```python
from build123d import *

# Parameters (mm, degrees)
SK_OUTPUT_PLATE_W        = 120.5
SK_OUTPUT_PLATE_H        = 93.5
SK_OUTPUT_PLATE_R        = 1.7
SK_OUTPUT_PLATE_R_2      = 5
OUTPUT_PLATE_DEPTH       = 5
SK_PITCH_PILOT_RECESS_R  = 15.15
PITCH_PILOT_RECESS_DEPTH = 2.2
SK_REAR_PLATE_W          = 93.5
SK_REAR_PLATE_H          = 86.75
SK_REAR_PLATE_R          = 8
SK_REAR_PLATE_R_2        = 1.7
REAR_PLATE_DEPTH         = 5
SK_TOP_PLATE_W           = 45.5
SK_TOP_PLATE_H           = 86.75
TOP_PLATE_DEPTH          = 5
SK_BOTTOM_PLATE_W        = 45.5
SK_BOTTOM_PLATE_H        = 86.75
BOTTOM_PLATE_DEPTH       = 5


with BuildPart() as part:
    # SK_Output_Plate → Output_Plate (new body)
    with BuildSketch(Plane(origin=(0, 0, 0), x_dir=(1, 0, 0), z_dir=(0, 1, 0))):
        with Locations((-30.25, 0)):
            Rectangle(SK_OUTPUT_PLATE_W, SK_OUTPUT_PLATE_H)
        with Locations(Location((20, 0, 0), (0, 0, 270))):
            Circle(SK_OUTPUT_PLATE_R, mode=Mode.SUBTRACT)
        with Locations(Location((10, 17.320508076, 0), (0, 0, 270))):
            Circle(SK_OUTPUT_PLATE_R, mode=Mode.SUBTRACT)
        with Locations(Location((-10, 17.320508076, 0), (0, 0, 270))):
            Circle(SK_OUTPUT_PLATE_R, mode=Mode.SUBTRACT)
        with Locations(Location((-20, 0, 0), (0, 0, 270))):
            Circle(SK_OUTPUT_PLATE_R, mode=Mode.SUBTRACT)
        with Locations(Location((-10, -17.320508076, 0), (0, 0, 270))):
            Circle(SK_OUTPUT_PLATE_R, mode=Mode.SUBTRACT)
        with Locations(Location((10, -17.320508076, 0), (0, 0, 270))):
            Circle(SK_OUTPUT_PLATE_R, mode=Mode.SUBTRACT)
        with Locations(Location((0, 0, 0), (0, 0, 270))):
            Circle(SK_OUTPUT_PLATE_R_2, mode=Mode.SUBTRACT)
    extrude(amount=OUTPUT_PLATE_DEPTH)

    # SK_Pitch_Pilot_Recess → Pitch_Pilot_Recess (cut)
    with BuildSketch(Plane(origin=(0, 0, 0), x_dir=(1, 0, 0), z_dir=(0, 1, 0))):
        with Locations(Location((0, 0, 0), (0, 0, 270))):
            Circle(SK_PITCH_PILOT_RECESS_R)
    extrude(amount=PITCH_PILOT_RECESS_DEPTH, mode=Mode.SUBTRACT)

    # SK_Rear_Plate → Rear_Plate (add)
    with BuildSketch(Plane(origin=(-90.5, 0, 0), x_dir=(0, 0, -1), z_dir=(1, 0, 0))):
        with Locations((0, 43.375)):
            Rectangle(SK_REAR_PLATE_W, SK_REAR_PLATE_H)
        with Locations((0, 45)):
            Circle(SK_REAR_PLATE_R, mode=Mode.SUBTRACT)
        with Locations((33, 45)):
            Circle(SK_REAR_PLATE_R_2, mode=Mode.SUBTRACT)
        with Locations((16.5, 73.578838325)):
            Circle(SK_REAR_PLATE_R_2, mode=Mode.SUBTRACT)
        with Locations((-16.5, 73.578838325)):
            Circle(SK_REAR_PLATE_R_2, mode=Mode.SUBTRACT)
        with Locations((-33, 45)):
            Circle(SK_REAR_PLATE_R_2, mode=Mode.SUBTRACT)
        with Locations((-16.5, 16.421161675)):
            Circle(SK_REAR_PLATE_R_2, mode=Mode.SUBTRACT)
        with Locations((16.5, 16.421161675)):
            Circle(SK_REAR_PLATE_R_2, mode=Mode.SUBTRACT)
    extrude(amount=REAR_PLATE_DEPTH)

    # SK_Top_Plate → Top_Plate (add)
    with BuildSketch(Plane.XY.offset(41.75)):
        with Locations((-67.75, 43.375)):
            Rectangle(SK_TOP_PLATE_W, SK_TOP_PLATE_H)
    extrude(amount=TOP_PLATE_DEPTH)

    # SK_Bottom_Plate → Bottom_Plate (add)
    with BuildSketch(Plane.XY.offset(-46.75)):
        with Locations((-67.75, 43.375)):
            Rectangle(SK_BOTTOM_PLATE_W, SK_BOTTOM_PLATE_H)
    extrude(amount=BOTTOM_PLATE_DEPTH)


solid = part.part
```
Design review of the part built by this model. Coordinates are the model's own, in mm. A direction names the side the tool comes from. Round coordinates to 2 decimals unless told otherwise and drop trailing zeros. Order: outer loops, then holes, each group sorted by start corner. A loop starts at its lowest first (then second) coordinate and runs counter-clockwise, first axis right, second up. Notation, with made-up numbers: (-18.5, 32.25) - (9.5, 32.25) arc R12 ccw to (9.5, 50.25) - close; hole circle Ø7 at (-12, 37). An arc over 180 degrees is marked (long way). One line per question, with ' | ' between items.
Item 1: Take a section at B-B, the plane x = 20. Write out the cut boundary in (y, z).
Checks:
outline: (0, -46.75) - (5, -46.75) - (5, -1.7) - (0, -1.7) - close; (0, 1.7) - (5, 1.7) - (5, 46.75) - (0, 46.75) - close
Item 2: Machinability: for faces 1 (the face through (-66, 46, 41.75)), 2 (the face through (-88, 43.5, 32.2)), 3 (the face through (4, 2.2, -4)), which of the approach directions +Z, -Z, +X, -X, +Y, -Y give a long, thin tool a straight path to every point of the face, cutting with its end or side? Answer none if there is none.
Checks:
face 1: +X, +Y | face 2: +X, -X | face 3: -Y
Item 3: Wall thickness on line 1 (X direction, y = 1.75, z = 0); line 2 (Z direction, x = -63, y = 31); line 3 (Y direction, x = -42, z = -37): over which ranges is each line inside the solid? List them lowest first. Write a range as [from, to].
Checks:
line 1: [-90.5, -21.7], [-18.3, -15.15], [15.15, 18.3], [21.7, 30] | line 2: [-46.75, -41.75], [41.75, 46.75] | line 3: [0, 5]
Item 4: Take a section at D-D, the plane x = 0. Write out the cut boundary in (y, z).
Checks:
outline: (0, -46.75) - (5, -46.75) - (5, -5) - (2.2, -5) - (2.2, -15.15) - (0, -15.15) - close; (0, 15.15) - (2.2, 15.15) - (2.2, 5) - (5, 5) - (5, 46.75) - (0, 46.75) - close
Item 5: Take a section at A-A, the plane z = -33. Write out the cut boundary in (x, y), then the cut area to 3 significant figures.
Checks:
outline: (-90.5, 0) - (30, 0) - (30, 5) - (-85.5, 5) - (-85.5, 43.3) - (-90.5, 43.3) - close; (-90.5, 46.7) - (-85.5, 46.7) - (-85.5, 86.75) - (-90.5, 86.75) - close | area: 994 mm²
Item 6: For P1, Ø4, axis at x = -19.5, z = 31.5, coming from the +Y side; P2, Ø6, axis at y = 12, z = 20.5, coming from the +X side; P3, Ø9, axis at x = 2, z = 2.5, coming from the -Y side, all flat-tipped, find the tip position at first contact; note any pin that passes through.
Checks:
P1: y = 5 | P2: x = -85.5 | P3: y = 2.2
Item 7: Take a section at C-C, the plane y = 25.5. Write out the cut boundary in (x, z), then the cut area to 4 significant figures.
Checks:
outline: (-90.5, -46.75) - (-45, -46.75) - (-45, -41.75) - (-85.5, -41.75) - (-85.5, 41.75) - (-45, 41.75) - (-45, 46.75) - (-90.5, 46.75) - close | area: 872.5 mm²
Item 8: Draft analysis for pull direction X (two halves, no side actions). For faces 4 (the face through (-45, 45, 44)), 5 (the face through (-14.79, 1.08, -3.28)), 6 (the face through (-66, 46, -41.75)), state which applies: +X half, -X half, draft (parallel to the pull), parting line (faces both ways), or undercut.
Checks:
face 4: +X half | face 5: undercut | face 6: draft
